Could you check a few things on this model? Use its own coordinates, in mm. A direction names the side the tool comes from. Round coordinates to 2 decimals unless told otherwise and drop trailing zeros. Order: outer loops, then holes, each group sorted by start corner. A loop starts at its lowest first (then second) coordinate and runs counter-clockwise, first axis right, second up.
```python
from build123d import *

# Parameters (mm, degrees)
BOSS_EXTRUDE2_DEPTH = 5
SKETCH7_R           = 1.5
CUT_EXTRUDE1_DEPTH  = 5
CUT_EXTRUDE2_DEPTH  = 5
SKETCH14_R          = 1.5
CUT_EXTRUDE3_DEPTH  = 161.15617378
SKETCH16_R          = 2
CUT_EXTRUDE4_DEPTH  = 161.15617378
CUT_EXTRUDE5_DEPTH  = 5


with BuildPart() as part:
    # Sketch1 → Boss-Extrude2 (new body)
    with BuildSketch(Plane(origin=(0, 0, 0), x_dir=(1, 0, 0), z_dir=(0, 1, 0))):
        with BuildLine():
            Line((-120, 100), (1.39320225, 100))
            ThreePointArc((1.39320225, 100), (24.368494305, 97.324898947), (46.1145618, 89.4427191))
            Line((46.1145618, 89.4427191), (116.708203932, 54.145898034))
            ThreePointArc((116.708203932, 54.145898034), (122.759762125, 48.615456851), (125, 40.729490169))
            Line((125, 40.729490169), (125, -40.729490169))
            ThreePointArc((125, -40.729490169), (122.759762125, -48.615456851), (116.708203932, -54.145898034))
            Line((116.708203932, -54.145898034), (46.1145618, -89.4427191))
            ThreePointArc((46.1145618, -89.4427191), (24.368494305, -97.324898947), (1.39320225, -100))
            Line((1.39320225, -100), (-120, -100))
            ThreePointArc((-120, -100), (-123.535533906, -98.535533906), (-125, -95))
            Line((-125, -95), (-125, 95))
            ThreePointArc((-125, 95), (-123.535533906, 98.535533906), (-120, 100))
        make_face()
    extrude(amount=-BOSS_EXTRUDE2_DEPTH)

    # Sketch7 → Cut-Extrude1 (cut)
    with BuildSketch(Plane(origin=(0, 0, 0), x_dir=(1, 0, 0), z_dir=(0, 1, 0))):
        with Locations(Location((-100, 50.003580751, 0), (0, 0, 270))):
            Circle(SKETCH7_R)
        with Locations(Location((-100, -49.996419249, 0), (0, 0, 270))):
            Circle(SKETCH7_R)
        with Locations(Location((25, 75.003580751, 0), (0, 0, 270))):
            Circle(SKETCH7_R)
        with Locations(Location((25, -74.996419249, 0), (0, 0, 270))):
            Circle(SKETCH7_R)
    extrude(amount=-CUT_EXTRUDE1_DEPTH, mode=Mode.SUBTRACT)

    # Sketch8 → Cut-Extrude2 (cut)
    with BuildSketch(Plane(origin=(0, 0, 0), x_dir=(1, 0, 0), z_dir=(0, 1, 0))):
        with BuildLine():
            Line((-96.1, 90.5), (-96.1, 76.5))
            ThreePointArc((-96.1, 76.5), (-94, 74.4), (-91.9, 76.5))
            Line((-91.9, 76.5), (-91.9, 90.5))
            ThreePointArc((-91.9, 90.5), (-94, 92.6), (-96.1, 90.5))
        make_face()
        with BuildLine():
            Line((-68.1, 90.5), (-68.1, 76.5))
            ThreePointArc((-68.1, 76.5), (-66, 74.4), (-63.9, 76.5))
            Line((-63.9, 76.5), (-63.9, 90.5))
            ThreePointArc((-63.9, 90.5), (-66, 92.6), (-68.1, 90.5))
        make_face()
        with BuildLine():
            Line((-87.000000572, 88.4), (-73, 88.4))
            ThreePointArc((-73, 88.4), (-70.9, 90.5), (-73, 92.6))
            Line((-73, 92.6), (-87, 92.6))
            ThreePointArc((-87, 92.6), (-89.100000572, 90.500000286), (-87.000000572, 88.4))
        make_face()
        with BuildLine():
            Line((-87, 74.4), (-73, 74.4))
            ThreePointArc((-73, 74.4), (-70.9, 76.5), (-73, 78.6))
            Line((-73, 78.6), (-87, 78.6))
            ThreePointArc((-87, 78.6), (-89.1, 76.5), (-87, 74.4))
        make_face()
        with BuildLine():
            Line((-87, -78.6), (-73, -78.6))
            ThreePointArc((-73, -78.6), (-70.9, -76.5), (-73, -74.4))
            Line((-73, -74.4), (-87, -74.4))
            ThreePointArc((-87, -74.4), (-89.1, -76.5), (-87, -78.6))
        make_face()
        with BuildLine():
            Line((-87, -92.6), (-73, -92.6))
            ThreePointArc((-73, -92.6), (-70.9, -90.5), (-73, -88.4))
            Line((-73, -88.4), (-87.000000572, -88.4))
            ThreePointArc((-87.000000572, -88.4), (-89.100000572, -90.500000286), (-87, -92.6))
        make_face()
        with BuildLine():
            Line((-63.9, -90.5), (-63.9, -76.5))
            ThreePointArc((-63.9, -76.5), (-66, -74.4), (-68.1, -76.5))
            Line((-68.1, -76.5), (-68.1, -90.5))
            ThreePointArc((-68.1, -90.5), (-66, -92.6), (-63.9, -90.5))
        make_face()
        with BuildLine():
            Line((-91.9, -90.5), (-91.9, -76.5))
            ThreePointArc((-91.9, -76.5), (-94, -74.4), (-96.1, -76.5))
            Line((-96.1, -76.5), (-96.1, -90.5))
            ThreePointArc((-96.1, -90.5), (-94, -92.6), (-91.9, -90.5))
        make_face()
    extrude(amount=-CUT_EXTRUDE2_DEPTH, mode=Mode.SUBTRACT)

    # Sketch14 → Cut-Extrude3 (cut, through all)
    with BuildSketch(Plane(origin=(0, 0, 0), x_dir=(1, 0, 0), z_dir=(0, 1, 0))):
        with Locations(Location((92, -56.993839984, 0), (0, 0, 270))):
            Circle(SKETCH14_R)
        with Locations(Location((92, 56.999582207, 0), (0, 0, 270))):
            Circle(SKETCH14_R)
    extrude(amount=-CUT_EXTRUDE3_DEPTH, mode=Mode.SUBTRACT)

    # Sketch16 → Cut-Extrude4 (cut, through all)
    with BuildSketch(Plane(origin=(0, 0, 0), x_dir=(1, 0, 0), z_dir=(0, 1, 0))):
        with Locations(Location((80.9, 15, 0), (0, 0, 270))):
            Circle(SKETCH16_R)
        with Locations(Location((105, 15, 0), (0, 0, 270))):
            Circle(SKETCH16_R)
        with Locations(Location((105, -15, 0), (0, 0, 90))):
            Circle(SKETCH16_R)
        with Locations(Location((80.9, -15, 0), (0, 0, 90))):
            Circle(SKETCH16_R)
    extrude(amount=-CUT_EXTRUDE4_DEPTH, mode=Mode.SUBTRACT)

    # Sketch17 → Cut-Extrude5 (cut)
    with BuildSketch(Plane(origin=(0, 0, 0), x_dir=(1, 0, 0), z_dir=(0, 1, 0))):
        with BuildLine():
            Line((-67.5, 12.5), (-67.5, -12.5))
            ThreePointArc((-67.5, -12.5), (-80, -25), (-92.5, -12.5))
            Line((-92.5, -12.5), (-92.5, 12.5))
            ThreePointArc((-92.5, 12.5), (-80, 25), (-67.5, 12.5))
        make_face()
    extrude(amount=-CUT_EXTRUDE5_DEPTH, mode=Mode.SUBTRACT)


solid = part.part
```
Q1. For faces 1 (the flat face through (-80, -2, -88.4)), 2 (the flat face through (2, 0, -1)), which set-ups out of +Z, -Z, +X, -X, +Y, -Y let a thin tool reach every point of the face, with its end or its side?
Q2. I need wall thicknesses on L1, parallel to Z at x = -100, y = -2.45; L2, parallel to Z at x = 106, y = -1.95; L3, parallel to X at y = -4.25, z = 8.5. Which ranges of each line are inside material? Lowest first, please.
Q3. We'd pull the mould along Z, two halves only. Please class faces 3 (the flat face through (-63.9, -2, 84)), 4 (the cylindrical face through (24.68, -2.46, 97.25)), 5 (the cylindrical face through (-124, -2, -98)): released by +Z, released by -Z, zero draft, split by the parting line, or undercut.
Q4. Imagine slicing it at A-A, the plane y = -2.9. State how many separate pieces and enclosed holes the cut face has, then the cut area to 3 significant figures.
Q5. For P1, Ø3.5, axis at x = 105, z = -15, coming from the -Y side; P2, Ø2.5, axis at y = -1.5, z = -83, coming from the +X side; P3, Ø1.5, axis at y = -2, z = 82, coming from the +X side; P4, Ø1.5, axis at y = -3.5, z = -83.5, coming from the +X side, each with a flat end and sliding along its axis, tell me the tip position at first contact or that it passes through.
Q6. Imagine slicing it at C-C, the plane z = 65. Please give me the cut outline in (x, y), then the cut area to 3 significant figures.
Q7. Imagine slicing it at B-B, the plane x = 53. Please give me the cut outline in (y, z).
Filled in:
1. face 1: +Y, -Y
1. face 2: +Z, -Z, +X, -X, +Y
2. L1: z = -100 to -51.5, -48.5 to 48.5, 51.5 to 100
2. L2: z = -59.5 to -16.73, -13.27 to 13.27, 16.73 to 59.5
2. L3: x = -125 to -92.5, -67.5 to 125
3. face 3: undercut
3. face 4: released by +Z
3. face 5: released by -Z
4. separate pieces: 1
4. enclosed holes: 19
4. area: 43,100 mm2
5. P1: passes through
5. P2: stops at x = 61.5
5. P3: stops at x = 62.5
5. P4: stops at x = 59.5
6. outline: (-125, -5) - (95, -5) - (95, 0) - (-125, 0) - close
6. area: 1,100 mm2
7. outline: (-5, -86) - (0, -86) - (0, 86) - (-5, 86) - close
